from build123d import *

# Parameters (mm, degrees)
PAD_DEPTH         = 44
SKETCH001_R       = 150
POCKET_DEPTH      = 44.001
POCKET_DEPTH_BACK = -24.001


with BuildPart() as part:
    # Sketch → Pad (new body, symmetric)
    with BuildSketch(Plane.YZ):
        Polygon((30, 0), (44, 62.614113), (42, 61.213698), (20, 5), (-10, 5), (-22, 16.400415), (-24, 15), (-20, 0), align=None)
    extrude(amount=PAD_DEPTH, both=True)

    # Sketch001 → Pocket (cut, two sides)
    with BuildSketch(Plane(origin=(0, 0, 0), x_dir=(0, 0, -1), z_dir=(0, -1, 0))) as pocket_sk:
        Circle(SKETCH001_R)
        Polygon((0, -20), (-61.614113, -44), (-62.614113, -44), (-62.614113, -42), (-5, -12.5), (-5, 12.5), (-62.614113, 42), (-62.614113, 44), (-61.614113, 44), (0, 20), align=None, mode=Mode.SUBTRACT)
    extrude(amount=-POCKET_DEPTH, mode=Mode.SUBTRACT)
    extrude(pocket_sk.sketch, amount=-POCKET_DEPTH_BACK, mode=Mode.SUBTRACT)


solid = part.part
Source: CAD feature listing. Evaluate the final solid. Frame: model axes, mm. A direction names the side the tool comes from. Give positions to 0.01 mm unless a question says otherwise; leave off trailing zeros. Write each loop counter-clockwise with the first axis right and the second up, starting at its lowest first coordinate (ties: lowest second). Pieces come first, ordered by that corner, then holes. Notation, with made-up numbers: (8.25, -9) - (62.25, -9) arc R32 cw to (62.25, 23) - close; hole circle Ø2 at (37, 68). An arc over 180 degrees is marked (long way). Write item = value, one per line. Start each with the question number.
Q1. Material intervals for probe 1 along Z at (x, y) = (14, -4.5); probe 2 along X at (y, z) = (-19.5, 13); probe 3 along X at (y, z) = (30, 26), sorted ascending.
Q2. Cut plane C-C, the plane y = 25. Return loops of the section in (x, z), then the cut area to 3 significant figures.
Q3. Cut plane A-A, the plane z = 24.5. Return loops of the section in (x, y), then the cut area to 3 significant figures.
Q4. Cut plane D-D, the plane x = -4.5. Return loops of the section in (y, z).
Q5. Draft query along X for faces 1 (the flat face through (-42.92, 43.01, 61.92)), 2 (the flat face through (-25.72, 24.79, 14.69)), 3 (the flat face through (25.834, 24.791, 14.977)), 4 (the flat face through (22.81, 31.06, 25.14)). Return one class per face: +X half, -X half, draft (parallel to the pull), parting line (faces both ways), or undercut.
Q6. Cut plane B-B, the plane z = 7. Return loops of the section in (x, y).
Q7. Pin query (flat end, axial travel): pin 1 Ø1.5 at (x, y) = (-2, 8.5) entering from +Z; pin 2 Ø1 at (x, y) = (-2.5, -5.5) entering from -Z; pin 3 Ø10 at (x, z) = (34, 53.5) entering from -Y. Return the tip coordinate at first contact, or that it passes through.
Q8. Reachability of faces 5 (the flat face through (0, 5, 0)), 6 (the flat face through (-26.938, 28.607, 26.992)), 7 (the flat face through (-21.9, -23, 15.7)), 8 (the flat face through (0, 5, 5)), 9 (the flat face through (-14.81, -18.46, 9.51)) from +Z, -Z, +X, -X, +Y, -Y: full face, straight path, thin tool, end or side. Return the list, or none.
Computed values:
q1.probe_1 = 0 to 5
q1.probe_2 = -25.06 to -16.6, 16.6 to 25.06
q1.probe_3 = -30.13 to -23.25, 23.25 to 30.13
q2.outline = (-26.92, 17.78) - (-20, 0) - (20, 0) - (26.92, 17.78) - (19.04, 17.78) - (12.5, 5) - (-12.5, 5) - (-19.04, 17.78) - close
q2.area = 431 mm²
q3.outline = (-29.54, 27.63) - (-22.48, 27.63) - (-22.48, 35.48) - (-29.54, 35.48) - close; (22.48, 27.63) - (29.54, 27.63) - (29.54, 35.48) - (22.48, 35.48) - close
q3.area = 111 mm²
q4.outline = (-21.33, 5) - (-20, 0) - (30, 0) - (31.12, 5) - close
q5.face_1 = draft
q5.face_2 = -X half
q5.face_3 = +X half
q5.face_4 = undercut
q6.outline = (-22.73, -21.87) - (-13.52, -21.87) - (-13.52, -12.11) - (-22.73, -12.11) - close; (-22.73, 20.78) - (-13.52, 20.78) - (-13.52, 31.57) - (-22.73, 31.57) - close; (13.52, -21.87) - (22.73, -21.87) - (22.73, -12.11) - (13.52, -12.11) - close; (13.52, 20.78) - (22.73, 20.78) - (22.73, 31.57) - (13.52, 31.57) - close
q7.pin_1 = 5
q7.pin_2 = 0
q7.pin_3 = 37.05
q8.face_5 = -Z, +X, -X, +Y, -Y
q8.face_6 = +Z, +X, -X
q8.face_7 = +Z, +X, -X, -Y
q8.face_8 = +Z
q8.face_9 = +Z, +Y, -Y
